from build123d import *

# Parameters (mm, degrees)
SCHIZZO2_R               = 5
TAGLIO_ESTRUSIONE1_DEPTH = 21
SMUSSO1_SIZE             = 1
RACCORDO1_R              = 0.3


with BuildPart() as part:
    # Schizzo1 → Rivoluzione1 (revolve)
    with BuildSketch(Plane.XY):
        Polygon((0, 0), (0, 11), (1, 11), (1, 8.75), (4, 8.75), (4, 11), (18, 11), (18, 8.75), (21, 8.75), (21, 11), (24, 11), (24, 0), align=None)
    revolve(axis=Axis((24, 0, 0), (-1, 0, 0)))

    # Schizzo2 → Taglio-Estrusione1 (cut)
    with BuildSketch(Plane(origin=(24, 0, 0), x_dir=(0, 0, -1), z_dir=(1, 0, 0))):
        with Locations(Location((0, 0, 0), (0, 0, 90))):
            Circle(SCHIZZO2_R)
    extrude(amount=-TAGLIO_ESTRUSIONE1_DEPTH, mode=Mode.SUBTRACT)

    # Smusso1
    smusso1_edges = [part.edges().sort_by_distance(p)[0] for p in [
        (0, -11, 0),
        (24, -11, 0),
    ]]
    chamfer(smusso1_edges, length=SMUSSO1_SIZE - 0.0001)  # a hair under: the kernel refuses the full size

    # Raccordo1
    raccordo1_edges = [part.edges().sort_by_distance(p)[0] for p in [
        (21, -8.75, 0),
        (18, -8.75, 0),
        (4, -8.75, 0),
        (1, -8.75, 0),
    ]]
    fillet(raccordo1_edges, radius=RACCORDO1_R)


solid = part.part
Part model, mm, in its own coordinate system. A direction names the side the tool comes from. Give positions to 0.01 mm unless a question says otherwise; leave off trailing zeros. Order: outer loops, then holes, each group sorted by start corner. A loop starts at its lowest first (then second) coordinate and runs counter-clockwise, first axis right, second up. Notation, with made-up numbers: (-7.75, 50) - (17.25, 50) arc R30 cw to (17.25, 84) - close; hole circle Ø2 at (56.5, -16). An arc over 180 degrees is marked (long way). Use a Markdown table: item, result.
1) Saw through at A-A on x = 19.25. List the corners of the cut face in (y, z), plus the area to 3 significant figures.
Checked values:
| item | result |
|---|---|
| outline | circle Ø17.5 at (0, 0); hole circle Ø10 at (0, 0) |
| area | 162 mm² |
2) Probe L1, parallel to Z at x = 7.75, y = 0; L2, parallel to Z at x = 19.5, y = 0; L3, parallel to X at y = -7.5, z = -7.5. List the from-to ranges inside material, lowest first. Write a range as from..to.
Checked values:
| item | result |
|---|---|
| L1 | -11..-5, 5..11 |
| L2 | -8.75..-5, 5..8.75 |
| L3 | 0.61..1, 4..18, 21..23.39 |
3) Two-plate mould, pull along X, no slides. Class faces 4 (the flat face through (24, 2, -5)), 5 (the flat face through (18, 2, 9)), 6 (the cylindrical face through (13.65, -1.08, -4.88)): +X half, -X half, draft (parallel to the pull), parting line (faces both ways), or undercut.
Checked values:
| item | result |
|---|---|
| face 4 | +X half |
| face 5 | undercut |
| face 6 | draft |
4) Flat gauge pins, fed straight in: P1, Ø3, axis at x = 11.5, z = 2, coming from the -Y side; P2, Ø1, axis at y = 2.5, z = -2, coming from the +X side. Where does each tip first touch, or does it go through?
Checked values:
| item | result |
|---|---|
| P1 | y = -10.99 |
| P2 | x = 3 |
5) 3-axis set-ups, long thin cutter, end or side, ignore diameter. For faces 1 (the flat face through (3, 0, 0)), 2 (the cylindrical face through (19.517, -6.944, 5.324)), 3 (the flat face through (0, 0, 0)): which of +Z, -Z, +X, -X, +Y, -Y reach the whole face in a straight line?
Checked values:
| item | result |
|---|---|
| face 1 | +X |
| face 2 | none |
| face 3 | +Z, -Z, -X, +Y, -Y |
6) Saw through at C-C on x = 9.75. List the corners of the cut face in (y, z).
Checked values:
| item | result |
|---|---|
| outline | circle Ø22 at (0, 0); hole circle Ø10 at (0, 0) |
7) Saw through at B-B on z = -9.5. Count the separate pieces of the cut face and the enclosed holes in it, plus the area to 3 significant figures.
Checked values:
| item | result |
|---|---|
| separate pieces | 3 |
| enclosed holes | 0 |
| area | 195 mm² |
